Source: CAD feature listing. Evaluate the final solid. Frame: model axes, mm. A direction names the side the tool comes from. Coordinates: 2 decimals unless noted, no trailing zeros. Loops run counter-clockwise (first coordinate to the right, second up) from the corner with the lowest first, then second, coordinate; pieces in that order, holes last. Notation, with made-up numbers: M 74,63.5 L 117,63.5 A21 cw 117,99.5 Z; hole C -10,39.5 d6. An arc over 180 degrees is marked long. One line per question, with ' | ' between items. Start each with the question number.
1. Section query C-C, the plane y = 5.25. Output: boundary loops of the cut face in (x, z) (1 decimal), and give its area (3 significant figures).
2. Section query B-B, the plane x = 0. Output: boundary loops of the cut face in (y, z).
3. Pin query (flat end, axial travel): P1, Ø1.2, axis at x = 3, y = 6, coming from the +Z side; P2, Ø5.5, axis at x = -0.5, z = 18, coming from the +Y side. Return the tip coordinate at first contact, or that it passes through.
4. Section query D-D, the plane z = 17.75. Output: boundary loops of the cut face in (x, y).
5. Access query for faces 5 (the flat face through (4, 4, 10)), 6 (the flat face through (-5, 3, 3)), 7 (the flat face through (0, 0, 10)), 8 (the flat face through (0, 4, 17)), 9 (the flat face through (-4, 4, 7)). Directions: +Z, -Z, +X, -X, +Y, -Y. A direction counts if a zero-diameter tool reaches every point of the face in a straight line with its end or side. Return the directions, or none.
6. Ray query, probe 1 along Z at (x, y) = (-2.75, 1.5); probe 2 along Z at (x, y) = (3, 9); probe 3 along Y at (x, z) = (4.5, 17). Return the intervals inside material, ascending.
7. Mould query, pull axis Z, two halves, no side actions, for faces 1 (the flat face through (2.5, 5, 8)), 2 (the flat face through (-2.5, 5, 8)), 3 (the flat face through (-5, 3, 14)), 4 (the flat face through (0, 2, 20)). Classes: pulls with the +Z half, pulls with the -Z half, needs draft (parallel to the pull), parting line crosses it, or undercut.
8. Section query A-A, the plane z = 3.5. Output: boundary loops of the cut face in (x, y), and give its area (3 significant figures).
```python
from build123d import *

# Parameters (mm, degrees)
F1_DEPTH = 20
F2_W     = 8
F2_H     = 5
F3_DEPTH = 25.4
F4_W     = 2.5
F4_H     = 3
F5_DEPTH = 38.1
F7_R     = 1.5875
F8_DEPTH = 25.4


with BuildPart() as f1:
    # F0 (on Top) → F1 (new body)
    with BuildSketch(Plane.XY):
        Polygon((0, 12), (0, 0), (5, 0), (5, 6.803848), (2, 12), align=None)
    extrude(amount=F1_DEPTH)

    # F2 (on face) → F3 (cut)
    with BuildSketch(Plane(origin=(0, 0, 0), x_dir=(0, -1, 0), z_dir=(-1, 0, 0))):
        with Locations((-8, 17.5)):
            Rectangle(F2_W, F2_H)
    extrude(amount=-F3_DEPTH, mode=Mode.SUBTRACT)

    # F4 (on face) → F5 (cut)
    with BuildSketch(Plane.XZ):
        with Locations((3.75, 8.5)):
            Rectangle(F4_W, F4_H)
    extrude(amount=-F5_DEPTH, mode=Mode.SUBTRACT)

    # F6: F1 across face


with BuildPart() as f1_1:
    add(f1.part)
    add(f1.part.mirror(Plane(origin=(0, 5.6, 8.5), x_dir=(0, -1, 0), z_dir=(-1, 0, 0))))

    # F7 (on face) → F8 (cut)
    with BuildSketch(Plane.XZ):
        with Locations((0, 3.5)):
            Circle(F7_R)
    extrude(amount=-F8_DEPTH, mode=Mode.SUBTRACT)


solid = f1_1.part
```
Taken from the geometry:
1) outline: M -5,0 L 5,0 L 5,7 L 2.5,7 L 2.5,10 L 5,10 L 5,15 L -5,15 L -5,10 L -2.5,10 L -2.5,7 L -5,7 Z; hole C 0,3.5 d3.2 | area: 127 mm^2
2) outline: M 0,0 L 12,0 L 12,1.91 L 0,1.91 Z; M 0,5.09 L 12,5.09 L 12,15 L 4,15 L 4,20 L 0,20 Z
3) P1: z = 15 | P2: y = 4
4) outline: M -5,0 L 5,0 L 5,4 L -5,4 Z
5) face 5: +X, +Y, -Y | face 6: +Z, -Z, -X, +Y, -Y | face 7: +Z, -Z, +X, -X, -Y | face 8: +Z, +X, -X, +Y | face 9: -X, +Y, -Y
6) probe 1: 0 to 7, 10 to 20 | probe 2: 0 to 7, 10 to 15 | probe 3: 0 to 4
7) face 1: undercut | face 2: undercut | face 3: needs draft | face 4: pulls with the +Z half
8) outline: M -5,0 L -1.59,0 L -1.59,12 L -2,12 L -5,6.8 Z; M 1.59,0 L 5,0 L 5,6.8 L 2,12 L 1.59,12 Z | area: 66.3 mm^2
